Model file for the job. Use its own axes, mm. A direction names the side the tool comes from. Give positions to 0.01 mm unless a question says otherwise; leave off trailing zeros. Loops run counter-clockwise (first coordinate to the right, second up) from the corner with the lowest first, then second, coordinate; pieces in that order, holes last. Notation, with made-up numbers: M 22,74 L 56,74 A23 cw 56,87 Z; hole C 20,-1.5 d4. An arc over 180 degrees is marked long. Answer in a Markdown table with one row per item.
```python
from build123d import *

# Parameters (mm, degrees)
BOSS_EXTRUDE1_DEPTH = 3


with BuildPart() as part:
    # Sketch1 → Boss-Extrude1 (new body)
    with BuildSketch(Plane.XY):
        with BuildLine():
            Line((-15.5, 27.693204924), (-8, 27.693204924))
            Line((-8, 27.693204924), (-7, 26.693204924))
            Line((-7, 26.693204924), (-7, 20.193204924))
            Line((-7, 20.193204924), (-4, 20.193204924))
            Line((-4, 20.193204924), (-4, 26.693204924))
            Line((-4, 26.693204924), (-3, 27.693204924))
            Line((-3, 27.693204924), (4.5, 27.693204924))
            Line((4.5, 27.693204924), (5.5, 26.693204924))
            Line((5.5, 26.693204924), (5.5, 20.193204924))
            Line((5.5, 20.193204924), (8.5, 20.193204924))
            Line((8.5, 20.193204924), (8.5, 26.693204924))
            Line((8.5, 26.693204924), (9.5, 27.693204924))
            Line((9.5, 27.693204924), (14.5, 27.693204924))
            ThreePointArc((14.5, 27.693204924), (18.035533906, 26.22873883), (19.5, 22.693204924))
            Line((19.5, 22.693204924), (19.5, 12.193204924))
            Line((19.5, 12.193204924), (18.5, 11.193204924))
            Line((18.5, 11.193204924), (12.5, 11.193204924))
            Line((12.5, 11.193204924), (12.5, 8.193204924))
            Line((12.5, 8.193204924), (18.5, 8.193204924))
            Line((18.5, 8.193204924), (19.5, 7.193204924))
            Line((19.5, 7.193204924), (19.5, -0.806795076))
            Line((19.5, -0.806795076), (18.5, -1.806795076))
            Line((18.5, -1.806795076), (12.5, -1.806795076))
            Line((12.5, -1.806795076), (12.5, -4.806795076))
            Line((12.5, -4.806795076), (18.5, -4.806795076))
            Line((18.5, -4.806795076), (19.5, -5.806795076))
            Line((19.5, -5.806795076), (19.5, -13.806795076))
            Line((19.5, -13.806795076), (18.5, -14.806795076))
            Line((18.5, -14.806795076), (12.5, -14.806795076))
            Line((12.5, -14.806795076), (12.5, -17.806795076))
            Line((12.5, -17.806795076), (18.5, -17.806795076))
            Line((18.5, -17.806795076), (19.5, -18.806795076))
            Line((19.5, -18.806795076), (19.5, -26.806795076))
            Line((19.5, -26.806795076), (18.5, -27.806795076))
            Line((18.5, -27.806795076), (12.5, -27.806795076))
            Line((12.5, -27.806795076), (12.5, -30.806795076))
            Line((12.5, -30.806795076), (18.5, -30.806795076))
            Line((18.5, -30.806795076), (19.5, -31.806795076))
            Line((19.5, -31.806795076), (19.5, -42.306795076))
            ThreePointArc((19.5, -42.306795076), (18.035533906, -45.842328982), (14.5, -47.306795076))
            Line((14.5, -47.306795076), (9.5, -47.306795076))
            Line((9.5, -47.306795076), (8.5, -46.306795076))
            Line((8.5, -46.306795076), (8.5, -39.806795076))
            Line((8.5, -39.806795076), (5.5, -39.806795076))
            Line((5.5, -39.806795076), (5.5, -46.306795076))
            Line((5.5, -46.306795076), (4.5, -47.306795076))
            Line((4.5, -47.306795076), (-3, -47.306795076))
            Line((-3, -47.306795076), (-4, -46.306795076))
            Line((-4, -46.306795076), (-4, -39.806795076))
            Line((-4, -39.806795076), (-7, -39.806795076))
            Line((-7, -39.806795076), (-7, -46.306795076))
            Line((-7, -46.306795076), (-8, -47.306795076))
            Line((-8, -47.306795076), (-15.5, -47.306795076))
            Line((-15.5, -47.306795076), (-16.5, -46.306795076))
            Line((-16.5, -46.306795076), (-16.5, -39.806795076))
            Line((-16.5, -39.806795076), (-19.5, -39.806795076))
            Line((-19.5, -39.806795076), (-19.5, -46.306795076))
            Line((-19.5, -46.306795076), (-20.5, -47.306795076))
            Line((-20.5, -47.306795076), (-25.5, -47.306795076))
            ThreePointArc((-25.5, -47.306795076), (-29.035533906, -45.842328982), (-30.5, -42.306795076))
            Line((-30.5, -42.306795076), (-30.5, -31.806795076))
            Line((-30.5, -31.806795076), (-29.5, -30.806795076))
            Line((-29.5, -30.806795076), (-23.5, -30.806795076))
            Line((-23.5, -30.806795076), (-23.5, -27.806795076))
            Line((-23.5, -27.806795076), (-29.5, -27.806795076))
            Line((-29.5, -27.806795076), (-30.5, -26.806795076))
            Line((-30.5, -26.806795076), (-30.5, -18.806795076))
            Line((-30.5, -18.806795076), (-29.5, -17.806795076))
            Line((-29.5, -17.806795076), (-23.5, -17.806795076))
            Line((-23.5, -17.806795076), (-23.5, -14.806795076))
            Line((-23.5, -14.806795076), (-29.5, -14.806795076))
            Line((-29.5, -14.806795076), (-30.5, -13.806795076))
            Line((-30.5, -13.806795076), (-30.5, -5.806795076))
            Line((-30.5, -5.806795076), (-29.5, -4.806795076))
            Line((-29.5, -4.806795076), (-23.5, -4.806795076))
            Line((-23.5, -4.806795076), (-23.5, -1.806795076))
            Line((-23.5, -1.806795076), (-29.5, -1.806795076))
            Line((-29.5, -1.806795076), (-30.5, -0.806795076))
            Line((-30.5, -0.806795076), (-30.5, 7.193204924))
            Line((-30.5, 7.193204924), (-29.5, 8.193204924))
            Line((-29.5, 8.193204924), (-23.5, 8.193204924))
            Line((-23.5, 8.193204924), (-23.5, 11.193204924))
            Line((-23.5, 11.193204924), (-29.5, 11.193204924))
            Line((-29.5, 11.193204924), (-30.5, 12.193204924))
            Line((-30.5, 12.193204924), (-30.5, 22.693204924))
            ThreePointArc((-30.5, 22.693204924), (-29.035533906, 26.22873883), (-25.5, 27.693204924))
            Line((-25.5, 27.693204924), (-20.5, 27.693204924))
            Line((-20.5, 27.693204924), (-19.5, 26.693204924))
            Line((-19.5, 26.693204924), (-19.5, 20.193204924))
            Line((-19.5, 20.193204924), (-16.5, 20.193204924))
            Line((-16.5, 20.193204924), (-16.5, 26.693204924))
            Line((-16.5, 26.693204924), (-15.5, 27.693204924))
        make_face()
    extrude(amount=BOSS_EXTRUDE1_DEPTH)


solid = part.part
```
Q1. Saw through at B-B (x = -18.5). Give the cut face in (y, z).
Reported:
| item | result |
|---|---|
| outline | M -39.81,0 L 20.19,0 L 20.19,3 L -39.81,3 Z |
Q2. Probe probe 1 along X at (y, z) = (-41, 0.75); probe 2 along Y at (x, z) = (-26, 1.95); probe 3 along Y at (x, z) = (17, 1.75). List the from-to ranges inside material, lowest first.
Reported:
| item | result |
|---|---|
| probe 1 | -30.5 to -19.5, -16.5 to -7, -4 to 5.5, 8.5 to 19.5 |
| probe 2 | -47.28 to -30.81, -27.81 to -17.81, -14.81 to -4.81, -1.81 to 8.19, 11.19 to 27.67 |
| probe 3 | -46.64 to -30.81, -27.81 to -17.81, -14.81 to -4.81, -1.81 to 8.19, 11.19 to 27.02 |
Q3. 3-axis set-ups, long thin cutter, end or side, ignore diameter. For faces 1 (the face through (-23.5, 10, 1)), 2 (the face through (12.5, -29, 1)), 3 (the face through (8.5, -43, 1)): which of +Z, -Z, +X, -X, +Y, -Y reach the whole face in a straight line?
Reported:
| item | result |
|---|---|
| face 1 | +Z, -Z, -X |
| face 2 | +Z, -Z, +X |
| face 3 | +Z, -Z, -Y |
Q4. Drop flat-ended pins along their axis: pin 1 (1.5 mm diameter, centred on y = 24, z = 1, fed in from -X); pin 2 (1.5 mm diameter, centred on x = -19.5, z = 1.5, fed in from +Y); pin 3 (1.5 mm diameter, centred on x = 6.5, z = 1.5, fed in from -Y). Give the stop position or say it passes through.
Reported:
| item | result |
|---|---|
| pin 1 | x = -30.47 |
| pin 2 | y = 27.44 |
| pin 3 | y = -39.81 |
Q5. Saw through at A-A (y = -16.5). Give the cut face in (x, z).
Reported:
| item | result |
|---|---|
| outline | M -23.5,0 L 12.5,0 L 12.5,3 L -23.5,3 Z |
